Verification items for the finished model (mm, model axes). Face numbers are marked on the shaded views. A direction names the side the tool comes from. Coordinates: 2 decimals unless noted, no trailing zeros. Loops run counter-clockwise (first coordinate to the right, second up) from the corner with the lowest first, then second, coordinate; pieces in that order, holes last.
Q1. Sectioned sample at D-D (z = 54.5). Enter the section's corners in (x, y), then the cut area to 3 significant figures.
Q2. Sectioned sample at A-A (y = 0). Enter the section's corners in (x, z), then the cut area to 4 significant figures.
Q3. Sectioned sample at C-C (z = 107). Enter the section's corners in (x, y), then the cut area to 3 significant figures.
Q4. Go/stop test with flat-tipped pins: P1, Ø4, axis at y = 26, z = 179, coming from the +X side; P2, Ø6, axis at x = -41, z = 134, coming from the -Y side; P3, Ø8, axis at y = -2.5, z = 50.5, coming from the +X side. Record where each tip stops, or that it passes through.
Q5. Sectioned sample at B-B (x = 13). Enter the section's corners in (y, z), then the cut area to 3 significant figures.
Q6. Material ranges on probe 1 along Z at (x, y) = (-30.5, -3.5); probe 2 along Z at (x, y) = (-49.5, -17); probe 3 along X at (y, z) = (-0.5, 28), recorded low to high.
Q7. Access from +Z, -Z, +X, -X, +Y, -Y to the whole of each face (thin tool, end or side, straight path). Record for the marked faces 1, 2 and 3.
```python
from build123d import *

# Parameters (mm, degrees)
ESBO_O1_R                = 30
RESSALTO_EXTRUS_O1_DEPTH = 30
ESBO_O2_R                = 45
RESSALTO_EXTRUS_O3_DEPTH = 45
ESBO_O3_R                = 55
RESSALTO_EXTRUS_O4_DEPTH = 80
ESBO_O4_R                = 35
RESSALTO_EXTRUS_O5_DEPTH = 50
ESBO_O5_R                = 20
RESSALTO_EXTRUS_O6_DEPTH = 45


with BuildPart() as part:
    # Esboço1 → Ressalto-extrusão1 (new body)
    with BuildSketch(Plane.XY):
        Circle(ESBO_O1_R)
    extrude(amount=RESSALTO_EXTRUS_O1_DEPTH)

    # Esboço2 → Ressalto-extrusão3 (add)
    with BuildSketch(Plane.XY.offset(30)):
        with Locations(Location((0, 0, 0), (0, 0, 180))):
            Circle(ESBO_O2_R)
    extrude(amount=RESSALTO_EXTRUS_O3_DEPTH)

    # Esboço3 → Ressalto-extrusão4 (add)
    with BuildSketch(Plane.XY.offset(75)):
        Circle(ESBO_O3_R)
    extrude(amount=RESSALTO_EXTRUS_O4_DEPTH)

    # Esboço4 → Ressalto-extrusão5 (add)
    with BuildSketch(Plane.XY.offset(155)):
        Circle(ESBO_O4_R)
    extrude(amount=RESSALTO_EXTRUS_O5_DEPTH)

    # Esboço5 → Ressalto-extrusão6 (add)
    with BuildSketch(Plane.XY.offset(205)):
        with Locations(Location((0, 0, 0), (0, 0, 180))):
            Circle(ESBO_O5_R)
    extrude(amount=RESSALTO_EXTRUS_O6_DEPTH)


solid = part.part
```
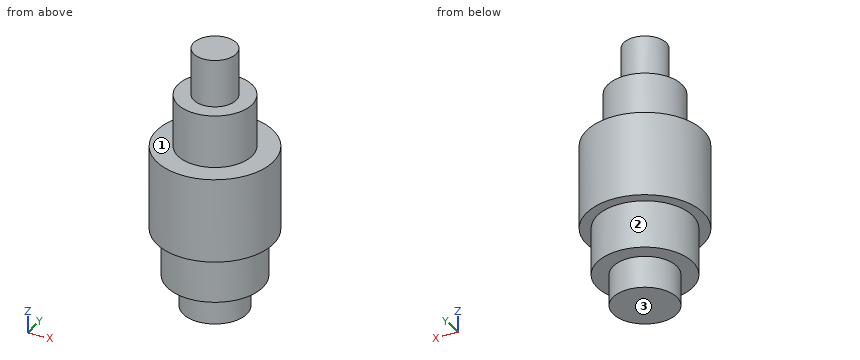
Geometry check:
1. outline: circle Ø90 at (0, 0)
1. area: 6,360 mm2
2. outline: (-55, 75) - (-45, 75) - (-45, 30) - (-30, 30) - (-30, 0) - (30, 0) - (30, 30) - (45, 30) - (45, 75) - (55, 75) - (55, 155) - (35, 155) - (35, 205) - (20, 205) - (20, 250) - (-20, 250) - (-20, 205) - (-35, 205) - (-35, 155) - (-55, 155) - close
2. area: 19,950 mm2
3. outline: circle Ø110 at (0, 0)
3. area: 9,500 mm2
4. P1: stops at x = 25.48
4. P2: stops at y = -39.76
4. P3: stops at x = 45
5. outline: (-53.44, 75) - (-43.08, 75) - (-43.08, 30) - (-27.04, 30) - (-27.04, 0) - (27.04, 0) - (27.04, 30) - (43.08, 30) - (43.08, 75) - (53.44, 75) - (53.44, 155) - (32.5, 155) - (32.5, 205) - (15.2, 205) - (15.2, 250) - (-15.2, 250) - (-15.2, 205) - (-32.5, 205) - (-32.5, 155) - (-53.44, 155) - close
5. area: 18,700 mm2
6. probe 1: z = 30 to 205
6. probe 2: z = 75 to 155
6. probe 3: x = -30 to 30
7. face 1: +Z
7. face 2: -Z
7. face 3: -Z, +X, -X, +Y, -Y
